Geometry check sheet. Reference: the model listing, model coordinates, mm. A direction names the side the tool comes from. Give positions to 0.01 mm unless a question says otherwise; leave off trailing zeros. Order: outer loops, then holes, each group sorted by start corner. A loop starts at its lowest first (then second) coordinate and runs counter-clockwise, first axis right, second up. Notation, with made-up numbers: M 56.5,79.5 L 103.5,79.5 A17 cw 103.5,102.5 Z; hole C 68,63.5 d7. An arc over 180 degrees is marked long. Use CSV: the item, a comma, the result in double quotes. Start each with the question number.
from build123d import *

# Parameters (mm, degrees)
F0_R     = 1.4
F1_DEPTH = 20
F3_DEPTH = 25


with BuildPart() as f1:
    # F0 (on Top) → F1 (new body)
    with BuildSketch(Plane.XY):
        with BuildLine():
            Line((-7.0003855483, -10.0099180601), (-6.7623309092, 3.5543028464))
            ThreePointArc((-6.7623309092, 3.5543028464), (-10.4585665785, 6.0054288438), (-10.3461336795, 1.5717468952))
            ThreePointArc((-10.3461336795, 1.5717468952), (-10.3233728773, 1.5610396555), (-10.3007163302, 1.5501135413))
            ThreePointArc((-10.3007163302, 1.5501135413), (-9.2560773016, 0.6249853883), (-8.8374101803, -0.706123413))
            ThreePointArc((-8.8374101803, -0.706123413), (-8.8362952804, -0.8408801673), (-8.8421380502, -0.9755148131))
            Line((-8.8421380502, -0.9755148131), (-8.9212343032, -5.4823753058))
            ThreePointArc((-8.9212343032, -5.4823753058), (-8.9185680619, -5.6331193754), (-8.9265222058, -5.7836770552))
            ThreePointArc((-8.9265222058, -5.7836770552), (-9.3628437334, -6.9014074118), (-10.3321539521, -7.6086098761))
            ThreePointArc((-10.3321539521, -7.6086098761), (-10.33956522, -7.6112390978), (-10.3469681809, -7.6138916189))
            ThreePointArc((-10.3469681809, -7.6138916189), (-10.9553516609, -11.9987700238), (-7.0003855483, -10.0099180601))
        make_face()
        with Locations((-9.5000006258, -9.9660493433)):
            Circle(F0_R, mode=Mode.SUBTRACT)
        with Locations((-9.248400609, 3.8178506564)):
            Circle(F0_R, mode=Mode.SUBTRACT)
        with BuildLine():
            ThreePointArc((-10.3007163302, 1.5501135413), (-10.3233728773, 1.5610396555), (-10.3461336795, 1.5717468952))
            ThreePointArc((-10.3461336795, 1.5717468952), (-10.323479421, 1.5608159761), (-10.3007163302, 1.5501135413))
        make_face()
        with BuildLine():
            ThreePointArc((-8.8421380502, -0.9755148131), (-8.8362952804, -0.8408801673), (-8.8374101803, -0.706123413))
            Line((-8.8374101803, -0.706123413), (-8.8421380502, -0.9755148131))
        make_face()
        with BuildLine():
            Line((-8.9212343032, -5.4823753058), (-8.9265222058, -5.7836770552))
            ThreePointArc((-8.9265222058, -5.7836770552), (-8.9185680619, -5.6331193754), (-8.9212343032, -5.4823753058))
        make_face()
    extrude(amount=F1_DEPTH)

    # F2 (on face) → F3 (cut)
    with BuildSketch(Plane(origin=(-8.822300232, 0.1548330356, 0), x_dir=(-0.0175474867, -0.999846031, 0), z_dir=(-0.999846031, 0.0175474867, 0))):
        with BuildLine():
            Line((5.939424578, 4.2884354293), (5.939424578, 15.7115645707))
            ThreePointArc((5.939424578, 15.7115645707), (3.4002568038, 18.2507323449), (0.8610890296, 15.7115645707))
            Line((0.8610890296, 15.7115645707), (0.8610890296, 4.2884354293))
            ThreePointArc((0.8610890296, 4.2884354293), (3.4002568038, 1.7492676551), (5.939424578, 4.2884354293))
        make_face()
    extrude(amount=-F3_DEPTH, mode=Mode.SUBTRACT)


solid = f1.part
(1) Sectioned sample at D-D on x = -11.15. Record the cut outline in (y, z), then the cut area to 3 significant figures.
(2) Sectioned sample at A-A on z = 13. Give the number of separate pieces and of enclosed holes in the cut face, then the cut area to 3 significant figures.
(3) Draft check along Y on faces 1 (the face through (-9.267, 0.642, 9.86)), 2 (the face through (-8, -3, 20)). Enter one of: +Y half, -Y half, draft (parallel to the pull), parting line (faces both ways), or undercut.
(4) Access from +Z, -Z, +X, -X, +Y, -Y to the whole of each face (thin tool, end or side, straight path). Record for faces 3 (the face through (-7.9, -3.21, 1.75)), 4 (the face through (-10.53, -9.02, 9.86)), 5 (the face through (-9.353, -6.888, 9.86)).
(5) Sectioned sample at B-B on x = -10. Record the cut outline in (y, z).
(6) Thickness scan on line 1 (Y direction, x = -8, z = 15.75); line 2 (Y direction, x = -8.6, z = 15.5); line 3 (Y direction, x = -8.6, z = 2.75). Record the ranges inside material, lowest first.
(7) Sectioned sample at C-C on y = -10.5. Record the cut outline in (x, z).
(8) Go/stop test with a flat-tipped pin: P1, Ø5, axis at y = -2, z = 18, coming from the -X side. Record where the tip stops, or that it passes through.
Responses:
1,outline,"M -11.84,0 L -8.09,0 L -8.09,20 L -11.84,20 Z; M 2.19,0 L 5.44,0 L 5.44,20 L 2.19,20 Z"
1,area,"140 mm2"
2,separate pieces,"2"
2,enclosed holes,"2"
2,area,"38.3 mm2"
3,face 1,"undercut"
3,face 2,"draft"
4,face 3,"none"
4,face 4,"+Z, -Z"
4,face 5,"+Z, -Z, -X"
5,outline,"M -12.42,0 L -11.27,0 L -11.27,20 L -12.42,20 Z; M -8.66,0 L -7.46,0 L -7.46,20 L -8.66,20 Z; M 1.38,0 L 2.64,0 L 2.64,20 L 1.38,20 Z; M 5,0 L 6.2,0 L 6.2,20 L 5,20 Z"
6,line 1,"-11.97 to -5.8, -0.72 to 3.18, 4.45 to 5.98"
6,line 2,"-12.3 to -11.04, -8.89 to -5.79, -0.71 to 2.58, 5.06 to 6.23"
6,line 3,"-12.3 to -11.04, -8.89 to -5.27, -1.23 to 2.58, 5.06 to 6.23"
7,outline,"M -11.94,0 L -10.79,0 L -10.79,20 L -11.94,20 Z; M -8.21,0 L -7.06,0 L -7.06,20 L -8.21,20 Z"
8,P1,"x = -9.18"
